```python
from build123d import *

# Parameters (mm, degrees)
SKETCH1_R           = 40
BOSS_EXTRUDE1_DEPTH = 40
SKETCH2_W           = 80
SKETCH2_H           = 2
CUT_EXTRUDE1_DEPTH  = 19
CUT_EXTRUDE2_START  = -3
SKETCH3_R           = 5.5
CUT_EXTRUDE2_DEPTH  = 118.717043198
SKETCH4_R           = 3
CUT_EXTRUDE3_DEPTH  = 64.5
LPATTERN1_COUNT     = 3
LPATTERN1_PITCH     = 25
SKETCH5_R           = 4.5
SKETCH5_R_2         = 2.1
SKETCH5_R_3         = 3.75
CUT_EXTRUDE4_DEPTH  = 24.5
CHAMFER1_SIZE       = 1


with BuildPart() as part:
    # Sketch1 → Boss-Extrude1 (new, symmetric)
    with BuildSketch(Plane(origin=(0, 0, 0), x_dir=(0, 0, -1), z_dir=(1, 0, 0))):
        with BuildLine():
            Line((-53, -25), (-43.301270189, -25))
            ThreePointArc((-43.301270189, -25), (0, -50), (43.301270189, -25))
            Line((43.301270189, -25), (53, -25))
            Line((53, -25), (53, 38))
            Line((53, 38), (74, 38))
            Line((74, 38), (74, 53))
            Line((74, 53), (-74, 53))
            Line((-74, 53), (-74, 38))
            Line((-74, 38), (-53, 38))
            Line((-53, 38), (-53, -25))
        make_face()
        Circle(SKETCH1_R, mode=Mode.SUBTRACT)
    extrude(amount=BOSS_EXTRUDE1_DEPTH, both=True)

    # Sketch2 → Cut-Extrude1 (cut)
    with BuildSketch(Plane(origin=(0, 0, -53), x_dir=(-1, 0, 0), z_dir=(0, 0, -1))):
        with Locations((0, 6.5)):
            Rectangle(SKETCH2_W, SKETCH2_H)
    extrude(amount=-CUT_EXTRUDE1_DEPTH, mode=Mode.SUBTRACT)

    # Sketch3 → Cut-Extrude2 (cut, through all)
    with BuildSketch(Plane.XZ.offset(25).offset(CUT_EXTRUDE2_START)):
        with Locations(Location((25.000000054, -43.3, 0), (0, 0, 180.013232088))):
            Circle(SKETCH3_R)
    cut_extrude2 = extrude(amount=CUT_EXTRUDE2_DEPTH, mode=Mode.SUBTRACT)

    # Sketch4 → Cut-Extrude3 (cut)
    with BuildSketch(Plane.XZ.offset(22)):
        with Locations(Location((25.000000054, -43.3, 0), (0, 0, 270))):
            Circle(SKETCH4_R)
    cut_extrude3 = extrude(amount=-CUT_EXTRUDE3_DEPTH, mode=Mode.SUBTRACT)

    # LPattern1: Cut-Extrude2, Cut-Extrude3 ×3
    with Locations(*[(-i * LPATTERN1_PITCH, 0, 0) for i in range(1, LPATTERN1_COUNT)]):
        add(cut_extrude2, mode=Mode.SUBTRACT)
        add(cut_extrude3, mode=Mode.SUBTRACT)

    # Sketch5 → Cut-Extrude4 (cut)
    with BuildSketch(Plane(origin=(0, 53, 0), x_dir=(1, 0, 0), z_dir=(0, 1, 0))):
        with Locations(Location((0, 0, 0), (0, 0, 270))):
            Circle(SKETCH5_R)
        with Locations(Location((-32, 62.5, 0), (0, 0, 270))):
            Circle(SKETCH5_R_2)
        with Locations(Location((-20, 62.5, 0), (0, 0, 270))):
            Circle(SKETCH5_R_3)
        with Locations(Location((32, 62.5, 0), (0, 0, 270))):
            Circle(SKETCH5_R_2)
        with Locations(Location((20, 62.5, 0), (0, 0, 270))):
            Circle(SKETCH5_R_3)
        with Locations(Location((32, -62.5, 0), (0, 0, 270))):
            Circle(SKETCH5_R_2)
        with Locations(Location((20, -62.5, 0), (0, 0, 270))):
            Circle(SKETCH5_R_3)
        with Locations(Location((-20, -62.5, 0), (0, 0, 270))):
            Circle(SKETCH5_R_3)
        with Locations(Location((-32, -62.5, 0), (0, 0, 270))):
            Circle(SKETCH5_R_2)
    extrude(amount=-CUT_EXTRUDE4_DEPTH, mode=Mode.SUBTRACT)

    # Chamfer1
    chamfer1_edges = [part.edges().sort_by_distance(p)[0] for p in [
        (40, -50, 0),
        (-40, 45.5, -74),
        (-40, 38, -63.5),
        (-40, -9.75, -53),
        (-40, -25, -48.150635095),
        (-40, -50, 0),
        (-40, -25, 48.150635095),
        (-40, 6.5, 53),
        (40, -25, -48.150635095),
        (40, -9.75, -53),
        (0, 38, 74),
        (0, 38, -74),
        (0, -25, -53),
        (0, -25, 53),
        (40, 38, -63.5),
        (40, 45.5, -74),
        (40, 45.5, 74),
        (40, 38, 63.5),
        (-40, 22.75, -53),
        (40, 22.75, -53),
        (40, 6.5, 53),
        (40, -25, 48.150635095),
        (-40, 38, 63.5),
        (-40, 45.5, 74),
    ]]
    chamfer(chamfer1_edges, length=CHAMFER1_SIZE)


solid = part.part
```
Geometry check sheet. Reference: the model listing, model coordinates, mm. A direction names the side the tool comes from. Coordinates: 2 decimals unless noted, no trailing zeros. Order: outer loops, then holes, each group sorted by start corner. A loop starts at its lowest first (then second) coordinate and runs counter-clockwise, first axis right, second up.
Q1. Sectioned sample at C-C on y = -1. Record the cut outline in (x, z), and give its area (3 significant figures).
Reply:
outline: (-40, -52) - (-39, -53) - (39, -53) - (40, -52) - (40, -39.99) - (-40, -39.99) - close; (-40, 39.99) - (40, 39.99) - (40, 52) - (39, 53) - (-39, 53) - (-40, 52) - close; hole circle Ø6 at (-25, -43.3); hole circle Ø6 at (0, -43.3); hole circle Ø6 at (25, -43.3)
area: 2,000 mm2
Q2. Sectioned sample at B-B on x = 0. Give the number of separate pieces and of enclosed holes in the cut face, and give its area (3 significant figures).
Reply:
separate pieces: 3
enclosed holes: 0
area: 4,830 mm2
Q3. Sectioned sample at D-D on z = -62.5. Record the cut outline in (x, y).
Reply:
outline: (-40, 39) - (-39, 38) - (-34.1, 38) - (-34.1, 53) - (-40, 53) - close; (-29.9, 38) - (-23.75, 38) - (-23.75, 53) - (-29.9, 53) - close; (-16.25, 38) - (16.25, 38) - (16.25, 53) - (-16.25, 53) - close; (23.75, 38) - (29.9, 38) - (29.9, 53) - (23.75, 53) - close; (34.1, 38) - (39, 38) - (40, 39) - (40, 53) - (34.1, 53) - close
Q4. Tool access check on faces 1 (the face through (1, 23, -53)), 2 (the face through (1, 7, 53)), 3 (the face through (-32.8, 45.6, 64.44)), 4 (the face through (25.9, -8.44, -46.16)), 5 (the face through (39.84, -49.154, 0.729)). Record the directions out of +Z, -Z, +X, -X, +Y, -Y that give a thin tool (end or side, any length) a straight path to the whole face; none if there is none.
Reply:
face 1: -Z, +X, -X, -Y
face 2: +Z, +X, -X, -Y
face 3: +Y, -Y
face 4: -Y
face 5: +X, -Y
Q5. Sectioned sample at A-A on z = 0. Record the cut outline in (x, y), and give its area (3 significant figures).
Reply:
outline: (-40, -49) - (-39, -50) - (39, -50) - (40, -49) - (40, -40) - (-40, -40) - close; (-40, 40) - (-4.5, 40) - (-4.5, 53) - (-40, 53) - close; (4.5, 40) - (40, 40) - (40, 53) - (4.5, 53) - close
area: 1,720 mm2
Q6. Depth check by flat-ended pin: pin 1 Ø3.5 at (x, z) = (-25, -43.3) entering from -Y; pin 2 Ø7 at (x, z) = (20, 62.5) entering from -Y; pin 3 Ø10 at (x, z) = (10.5, 63.5) entering from -Y; pin 4 Ø9 at (x, z) = (26.5, -41.5) entering from -Y. Enter the tip coordinate at first touch or a pass-through.
Reply:
pin 1: stops at y = 42.5
pin 2: passes through
pin 3: stops at y = 38
pin 4: stops at y = -33.63
Q7. Thickness scan on probe 1 along X at (y, z) = (-7, -43.3); probe 2 along X at (y, z) = (47, 62.5); probe 3 along Z at (x, y) = (-17, 1). Record the ranges inside material, lowest first.
Reply:
probe 1: x = -40 to -28, -22 to -3, 3 to 22, 28 to 40
probe 2: x = -40 to -34.1, -29.9 to -23.75, -16.25 to 16.25, 23.75 to 29.9, 34.1 to 40
probe 3: z = -53 to -39.99, 39.99 to 53
Q8. Draft check along Z on faces 6 (the face through (1, 46, 74)), 7 (the face through (-33.863, 45.605, -61.531)), 8 (the face through (9, 53, -1)). Enter one of: released by +Z, released by -Z, zero draft, split by the parting line, or undercut.
Reply:
face 6: released by +Z
face 7: undercut
face 8: zero draft
